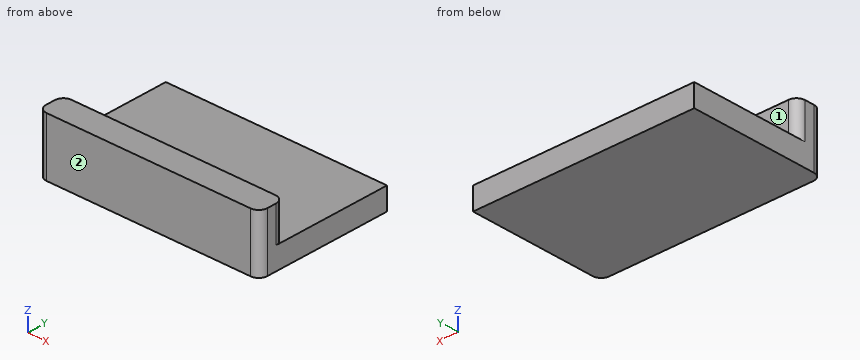
from build123d import *

# Parameters (mm, degrees)
SKETCH002_W  = 10
SKETCH002_H  = 1.2
PAD002_DEPTH = 1.6
SKETCH003_W  = 10
SKETCH003_H  = 6.2
PAD003_DEPTH = 1
FILLET001_R  = 0.39


with BuildPart() as part:
    # Sketch002 → Pad002 (new body)
    with BuildSketch(Plane.XY):
        with Locations((5, -0.6)):
            Rectangle(SKETCH002_W, SKETCH002_H)
    extrude(amount=PAD002_DEPTH)

    # Sketch003 → Pad003 (join)
    with BuildSketch(Plane.XY):
        with Locations((5, 1.9)):
            Rectangle(SKETCH003_W, SKETCH003_H)
    extrude(amount=-PAD003_DEPTH)

    # Fillet001
    fillet001_edges = [part.edges().sort_by_distance(p)[0] for p in [
        (0, -1.2, 0.3),
        (10, -1.2, 0.3),
        (10, 0, 0.8),
        (0, 0, 0.8),
    ]]
    fillet(fillet001_edges, radius=FILLET001_R)


solid = part.part
Can you work these out from the model? Positions are in its coordinate system, mm. Face numbers are marked on the shaded views. A direction names the side the tool comes from. Give positions to 0.01 mm unless a question says otherwise; leave off trailing zeros. Loops run counter-clockwise (first coordinate to the right, second up) from the corner with the lowest first, then second, coordinate; pieces in that order, holes last. Notation, with made-up numbers: (12, 7) -> (40, 7) arc R22 cw to (40, 25) -> close; hole circle Ø8 at (70.5, 10). An arc over 180 degrees is marked (long way). Return JSON: item names as keys, results as strings.
Q1. For pin 1 Ø1.6 at (x, y) = (6, 2.5) entering from +Z; pin 2 Ø0.8 at (x, z) = (7, 0.5) entering from +Y, each with a flat end and sliding along its axis, tell me the tip position at first contact or that it passes through.
Checks:
{"pin 1": "stops at z = 0", "pin 2": "stops at y = 0"}
Q2. I want a section at B-B, the plane x = 7.25. List the corners of the cut face in (y, z) for me.
Checks:
{"outline": "(-1.2, -1) -> (5, -1) -> (5, 0) -> (0, 0) -> (0, 1.6) -> (-1.2, 1.6) -> close"}
Q3. I need wall thicknesses on probe 1 along Z at (x, y) = (5.75, 4); probe 2 along Y at (x, z) = (8, 0.35). Which ranges of each line are inside material? Lowest first, please.
Checks:
{"probe 1": "z = -1 to 0", "probe 2": "y = -1.2 to 0"}
Q4. I want a section at A-A, the plane z = 1.1. List the corners of the cut face in (x, y) for me.
Checks:
{"outline": "(0, -0.81) arc R0.39 ccw to (0.39, -1.2) -> (9.61, -1.2) arc R0.39 ccw to (10, -0.81) -> (10, -0.39) arc R0.39 ccw to (9.61, 0) -> (0.39, 0) arc R0.39 ccw to (0, -0.39) -> close"}
Q5. On a 3-axis mill with a long thin cutter (end or side, diameter ignored), from which of +Z, -Z, +X, -X, +Y, -Y can I reach the whole of each face in a straight line? I mean the marked faces 1 and 2. Say none if no direction works.
Checks:
{"face 1": "+Z, +X, -X, +Y", "face 2": "+Z, -Z, +X, -X, -Y"}
Q6. I want a section at C-C, the plane y = 4.25. List the corners of the cut face in (x, z) for me, then the cut area to 3 significant figures.
Checks:
{"outline": "(0, -1) -> (10, -1) -> (10, 0) -> (0, 0) -> close", "area": "10.0 mm2"}
